Source: three-view drawing plus pictorial views. Frame: mm from the lowest corner of the part. Give positions to 0.01 mm unless a question says otherwise; leave off trailing zeros. Loops run counter-clockwise (first coordinate to the right, second up) from the corner with the lowest first, then second, coordinate; pieces in that order, holes last. Notation, with made-up numbers: (29.5, 24) -> (75.5, 24) arc R17 ccw to (75.5, 34) -> close; hole circle Ø5 at (22, 89.5). An arc over 180 degrees is marked (long way). Put each result on its own line as item: value.
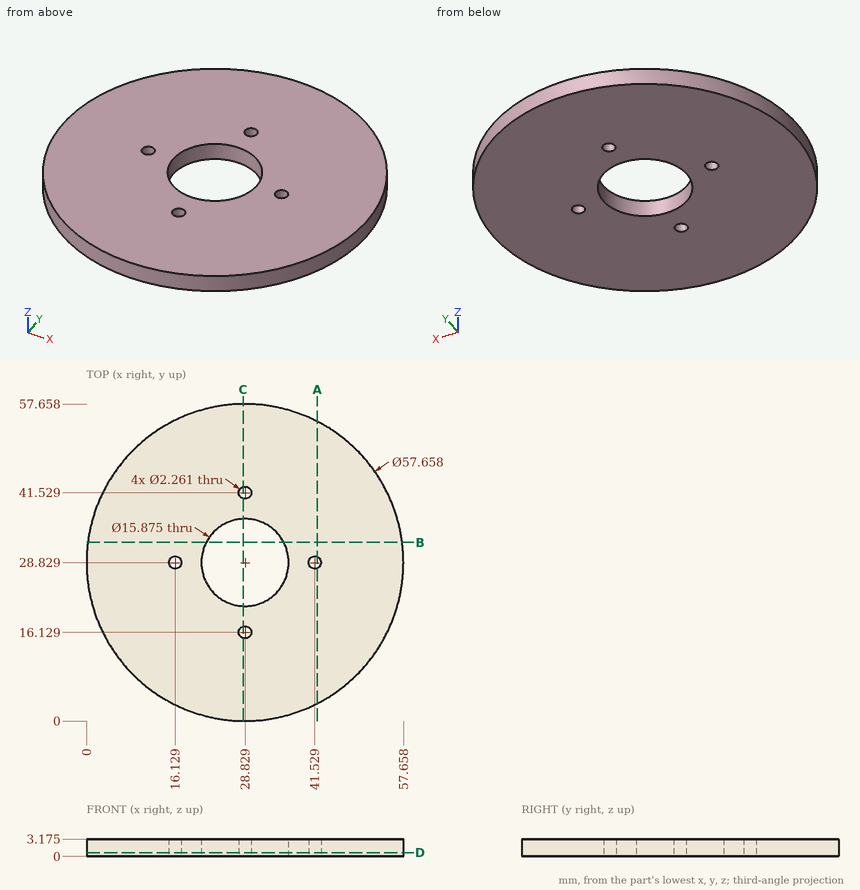
(1) First-contact query: P1, Ø1.5, axis at x = 27, z = 0.5, coming from the -Y side; P2, Ø2, axis at x = 41.529, y = 28.829, coming from the -Z side; P3, Ø1.5, axis at x = 49.5, z = 1, coming from the +Y side. Flat tips, straight axial feed; report the tip coordinate or a pass-through.
Calculated:
P1: stops at y = 0.02
P2: passes through
P3: stops at y = 49.67
(2) Section A-A on x = 42. Return loops of the section in (y, z) (1 decimal), then the cut area to 3 significant figures.
Calculated:
outline: (3.2, 0) -> (27.8, 0) -> (27.8, 3.2) -> (3.2, 3.2) -> close; (29.9, 0) -> (54.5, 0) -> (54.5, 3.2) -> (29.9, 3.2) -> close
area: 156 mm²
(3) Line query: probe 1 along Y at (x, z) = (35.5, 1.65) (1 decimal); probe 2 along X at (y, z) = (22, 2.8) (1 decimal); probe 3 along Y at (x, z) = (25.5, 0.85) (1 decimal). Output: solid intervals per line, ascending. Write a range as from..to.
Calculated:
probe 1: y = 0.8..24.5, 33.1..56.9
probe 2: x = 0.8..24.8, 32.9..56.8
probe 3: y = 0.2..21.6, 36..57.5
(4) Section B-B on y = 32.5. Return loops of the section in (x, z) (1 decimal), then the cut area to 3 significant figures.
Calculated:
outline: (0.2, 0) -> (21.8, 0) -> (21.8, 3.2) -> (0.2, 3.2) -> close; (35.9, 0) -> (57.4, 0) -> (57.4, 3.2) -> (35.9, 3.2) -> close
area: 137 mm²
(5) Section D-D on z = 0.7. Return loops of the section in (x, y) (1 decimal), then the cut area to 3 significant figures.
Calculated:
outline: circle Ø57.7 at (28.8, 28.8); hole circle Ø2.3 at (16.1, 28.8); hole circle Ø15.9 at (28.8, 28.8); hole circle Ø2.3 at (28.8, 16.1); hole circle Ø2.3 at (28.8, 41.5); hole circle Ø2.3 at (41.5, 28.8)
area: 2,400 mm²
(6) Section C-C on x = 28.5. Return loops of the section in (y, z) (1 decimal), then the cut area to 3 significant figures.
Calculated:
outline: (0, 0) -> (15, 0) -> (15, 3.2) -> (0, 3.2) -> close; (17.2, 0) -> (20.9, 0) -> (20.9, 3.2) -> (17.2, 3.2) -> close; (36.8, 0) -> (40.4, 0) -> (40.4, 3.2) -> (36.8, 3.2) -> close; (42.6, 0) -> (57.7, 0) -> (57.7, 3.2) -> (42.6, 3.2) -> close
area: 119 mm²
